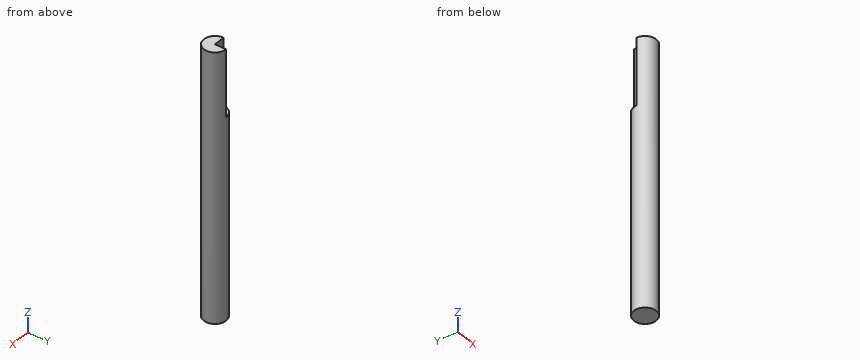
```python
from build123d import *

# Parameters (mm, degrees)
F0_R     = 12.7
F1_DEPTH = 304.8
F3_DEPTH = 76.2
F5_DEPTH = 76.2


with BuildPart() as f1:
    # F0 (on Top) → F1 (new body)
    with BuildSketch(Plane.XY):
        with Locations((-10.884415, 9.929642)):
            Circle(F0_R)
    extrude(amount=F1_DEPTH)

    # F2 (on face) → F3 (cut)
    with BuildSketch(Plane.XY.offset(304.8)):
        with BuildLine():
            ThreePointArc((1.815585, 9.929642), (1.714362, 11.529897), (1.412307, 13.104642))
            Line((1.412307, 13.104642), (-4.937693, 13.104642))
            Line((-4.937693, 13.104642), (-4.937693, 6.754642))
            Line((-4.937693, 6.754642), (1.412307, 6.754642))
            ThreePointArc((1.412307, 6.754642), (1.714362, 8.329388), (1.815585, 9.929642))
        make_face()
    extrude(amount=F3_DEPTH, mode=Mode.SUBTRACT)

    # F4 (on face) → F5 (cut)
    with BuildSketch(Plane.XY.offset(304.8)):
        with BuildLine():
            Line((-23.584415, 9.929642), (-10.884415, 9.929642))
            Line((-10.884415, 9.929642), (-10.884415, 22.629642))
            ThreePointArc((-10.884415, 22.629642), (-19.864671, 18.909898), (-23.584415, 9.929642))
        make_face()
    extrude(amount=-F5_DEPTH, mode=Mode.SUBTRACT)


solid = f1.part
```
Build history of the part. All positions in model axes, mm. Round coordinates to 2 decimals unless told otherwise and drop trailing zeros. Order: outer loops, then holes, each group sorted by start corner. A loop starts at its lowest first (then second) coordinate and runs counter-clockwise, first axis right, second up. Notation, with made-up numbers: (2.5, 28) - (44.5, 28) arc R22 ccw to (44.5, 41) - close; hole circle Ø10 at (85.25, 45.5). An arc over 180 degrees is marked (long way). Use a Markdown table: item, result.
1) Saw through at C-C on x = -14.5. Write the cut outline in (y, z).
Recorded:
| item | result |
|---|---|
| outline | (-2.24, 0) - (22.1, 0) - (22.1, 228.6) - (9.93, 228.6) - (9.93, 304.8) - (-2.24, 304.8) - close |
2) Wall check: L1, parallel to X at y = 10.25, z = 261.5; L2, parallel to X at y = 10.5, z = 106; L3, parallel to Z at x = -21.5, y = 15.75. Give the ranges that are in metal, low to high.
Recorded:
| item | result |
|---|---|
| L1 | x = -10.88 to 1.81 |
| L2 | x = -23.57 to 1.8 |
| L3 | z = 0 to 228.6 |
3) Saw through at B-B on y = 19. Write the cut outline in (x, z), and give its area (3 significant figures).
Recorded:
| item | result |
|---|---|
| outline | (-19.77, 0) - (-2, 0) - (-2, 304.8) - (-10.88, 304.8) - (-10.88, 228.6) - (-19.77, 228.6) - close |
| area | 4,740 mm² |
4) Saw through at D-D on z = 78.5. Write the cut outline in (x, y), and give its area (3 significant figures).
Recorded:
| item | result |
|---|---|
| outline | circle Ø25.4 at (-10.88, 9.93) |
| area | 507 mm² |
5) Flat gauge pins, fed straight in: pin 1 Ø4 at (y, z) = (13.5, 271.5) entering from -X; pin 2 Ø8 at (y, z) = (6, 250.5) entering from +X; pin 3 Ø4 at (y, z) = (1, 123.5) entering from +X; pin 4 Ø8 at (x, y) = (-21, 15) entering from +Z. Where does each tip first touch, or does it go through?
Recorded:
| item | result |
|---|---|
| pin 1 | stops at x = -10.88 |
| pin 2 | stops at x = 1.82 |
| pin 3 | stops at x = -0.24 |
| pin 4 | stops at z = 228.6 |
6) Saw through at A-A on z = 253. Write the cut outline in (x, y).
Recorded:
| item | result |
|---|---|
| outline | (-23.58, 9.93) arc R12.7 ccw (long way) to (-10.88, 22.63) - (-10.88, 9.93) - close |
